```python
from build123d import *

# Parameters (mm, degrees)
F0_W     = 25.4
F0_H     = 787.4
F1_DEPTH = 711.2
F2_W     = 25.4
F2_H     = 787.4
F3_DEPTH = 25.4
F4_W     = 25.4
F4_H     = 520.7
F5_DEPTH = 711.2
F8_DEPTH = 25.4


with BuildPart() as f1:
    # F0 (on Top) → F1 (new body)
    with BuildSketch(Plane.XY):
        with Locations((12.7, -393.7)):
            Rectangle(F0_W, F0_H)
    extrude(amount=F1_DEPTH)

    # F2 (on face) → F3 (join)
    with BuildSketch(Plane.XY.offset(711.2)):
        with BuildLine():
            Line((1562.1, 0), (25.4, 0))
            Line((25.4, 0), (25.4, -787.4))
            Line((25.4, -787.4), (520.7, -787.4))
            ThreePointArc((520.7, -787.4), (1022.965212, -582.066542), (1562.1, -520.7))
            Line((1562.1, -520.7), (1562.1, 0))
        make_face()
        with Locations((12.7, -393.7)):
            Rectangle(F2_W, F2_H)
    extrude(amount=F3_DEPTH)

    # F4 (on Top) → F5 (join)
    with BuildSketch(Plane.XY):
        with Locations((1549.4, -260.35)):
            Rectangle(F4_W, F4_H)
    extrude(amount=F5_DEPTH)

    # F7 (on offset) → F8 (join)
    with BuildSketch(Plane.XZ.offset(127)):
        with BuildLine():
            Line((25.4, 673.1), (25.4, 330.2))
            Line((25.4, 330.2), (1536.7, 330.2))
            Line((1536.7, 330.2), (1536.7, 673.1))
            Line((1536.7, 673.1), (1155.7, 673.1))
            ThreePointArc((1155.7, 673.1), (1078.855779, 682.776021), (1006.809008, 711.2))
            Line((1006.809008, 711.2), (555.290992, 711.2))
            ThreePointArc((555.290992, 711.2), (483.244221, 682.776021), (406.4, 673.1))
            Line((406.4, 673.1), (25.4, 673.1))
        make_face()
    extrude(amount=F8_DEPTH)


solid = f1.part
```
For this review, take the finished solid that the model builds, in its own axes (mm). A direction names the side the tool comes from. Give positions to 0.01 mm unless a question says otherwise; leave off trailing zeros. Write each loop counter-clockwise with the first axis right and the second up, starting at its lowest first coordinate (ties: lowest second). Pieces come first, ordered by that corner, then holes. Notation, with made-up numbers: M 25,-29.5 L 55,-29.5 A30 cw 55,3.5 Z; hole C 65,86.25 d5. An arc over 180 degrees is marked long. Answer as CSV lines item,"result".
1. Consider section C-C, the plane z = 382.5. Write out the cut boundary in (x, y), then the cut area to 3 significant figures.
Findings:
outline,"M 0,-787.4 L 25.4,-787.4 L 25.4,-152.4 L 1536.7,-152.4 L 1536.7,-520.7 L 1562.1,-520.7 L 1562.1,0 L 1536.7,0 L 1536.7,-127 L 25.4,-127 L 25.4,0 L 0,0 Z"
area,"71,600 mm2"
2. Wall thickness on line 1 (X direction, y = -339, z = 440); line 2 (Z direction, x = 470, y = -107.5); line 3 (Y direction, x = 170, z = 450): over which ranges is each line inside the solid? List them lowest first.
Findings:
line 1,"x = 0 to 25.4, 1536.7 to 1562.1"
line 2,"z = 711.2 to 736.6"
line 3,"y = -152.4 to -127"
3. Consider section D-D, the plane y = -308.5. Write out the cut boundary in (x, z), then the cut area to 3 significant figures.
Findings:
outline,"M 0,0 L 25.4,0 L 25.4,711.2 L 1536.7,711.2 L 1536.7,0 L 1562.1,0 L 1562.1,736.6 L 0,736.6 Z"
area,"75,800 mm2"
4. Consider section B-B, the plane x = 1266. Write out the cut boundary in (y, z).
Findings:
outline,"M -535.77,711.2 L 0,711.2 L 0,736.6 L -535.77,736.6 Z; M -152.4,330.2 L -127,330.2 L -127,673.1 L -152.4,673.1 Z"
5. Consider section A-A, the plane z = 96.5. Write out the cut boundary in (x, y), then the cut area to 3 significant figures.
Findings:
outline,"M 0,-787.4 L 25.4,-787.4 L 25.4,0 L 0,0 Z; M 1536.7,-520.7 L 1562.1,-520.7 L 1562.1,0 L 1536.7,0 Z"
area,"33,200 mm2"
6. For pin 1 (8 mm diameter, centred on x = 847.5, z = 333.5, fed in from -Y); pin 2 (6 mm diameter, centred on y = -595.5, z = 634.5, fed in from +X); pin 3 (12.5 mm diameter, centred on x = 969.5, y = -142, fed in from -Z); pin 4 (1 mm diameter, centred on y = -614.5, z = 513.5, fed in from -X), all flat-tipped, find the tip position at first contact; note any pin that passes through.
Findings:
pin 1,"stops at y = -152.4"
pin 2,"stops at x = 25.4"
pin 3,"stops at z = 330.2"
pin 4,"stops at x = 0"
7. For faces 5 (the flat face through (770, -152.4, 523)), 6 (the flat face through (770, -127, 523)), 7 (the flat face through (770, -301, 736.6)), list the 3-axis set-ups (+Z, -Z, +X, -X, +Y, -Y) from which the entire face can be reached by the end or side of a thin tool; tool diameter is ignored.
Findings:
face 5,"-Z, -Y"
face 6,"-Z, +Y"
face 7,"+Z, +X, -X, +Y, -Y"
8. Draft analysis for pull direction X (two halves, no side actions). For faces 1 (the flat face through (0, -399, 363)), 2 (the flat face through (430, 0, 721)), 3 (the flat face through (1536.7, -264, 351)), 4 (the cylindrical face through (484.3, -139.52, 683.05)), state which applies: +X half, -X half, draft (parallel to the pull), parting line (faces both ways), or undercut.
Findings:
face 1,"-X half"
face 2,"draft"
face 3,"undercut"
face 4,"undercut"
